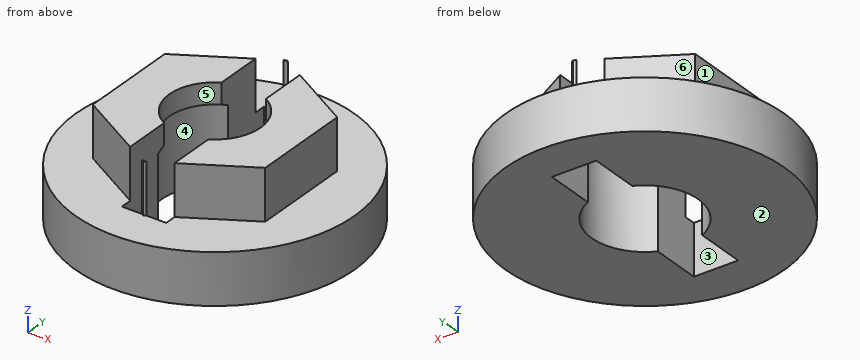
from build123d import *

# Parameters (mm, degrees)
F5_DEPTH  = 4
F4_R      = 5.5
F6_DEPTH  = 2
F7_W      = 1.75
F7_H      = 7.75
F8_DEPTH  = 5
F10_D     = 3.6
F11_D     = 4.2
F11_DEPTH = 3
F11_TIP   = 1.2618073


with BuildPart() as f5:
    # F4 (on Top) → F5 (new body)
    with BuildSketch(Plane.XY):
        Polygon((3.4, -1.9629909152), (3.4, 1.9629909152), (0, 3.9259818305), (-3.4, 1.9629909152), (-3.4, -1.9629909152), (0, -3.9259818305), align=None)
    extrude(amount=F5_DEPTH)

    # F4 (on Top) → F6 (join)
    with BuildSketch(Plane.XY):
        Circle(F4_R)
        Polygon((0, 3.9259818305), (3.4, 1.9629909152), (3.4, -1.9629909152), (0, -3.9259818305), (-3.4, -1.9629909152), (-3.4, 1.9629909152), align=None, mode=Mode.SUBTRACT)
    extrude(amount=F6_DEPTH)

    # F7 (on Top) → F8 (cut)
    with BuildSketch(Plane.XY):
        Rectangle(F7_W, F7_H)
    extrude(amount=F8_DEPTH, mode=Mode.SUBTRACT)

    # F10 (through all)
    with Locations(Plane(origin=(0, 0, 0), x_dir=(1, 0, 0), z_dir=(0, 0, -1))):
        with Locations((0, 0)):
            Hole(F10_D / 2)

    # F11
    with Locations(Plane(origin=(0, 0, 0), x_dir=(1, 0, 0), z_dir=(0, 0, -1))):
        with Locations((0, 0)):
            Hole(F11_D / 2, depth=F11_DEPTH)
            with Locations((0, 0, -(F11_DEPTH + F11_TIP / 2))):  # 118° drill point
                Cone(0, F11_D / 2, F11_TIP, mode=Mode.SUBTRACT)


solid = f5.part
Work out the finished part from the listing and answer in its coordinate system (mm). Face numbers are marked on the shaded views. A direction names the side the tool comes from. Round coordinates to 2 decimals unless told otherwise and drop trailing zeros. Write each loop counter-clockwise with the first axis right and the second up, starting at its lowest first coordinate (ties: lowest second). Pieces come first, ordered by that corner, then holes.
1) The mould has two halves that part along X. Classify the marked faces 1, 2 and 3: pulls with the +X half, pulls with the -X half, needs draft (parallel to the pull), parting line crosses it, or undercut.
2) A tool of negligible diameter and unlimited length cuts with its end or side. For the marked faces 4, 5 and 6, from which of +Z, -Z, +X, -X, +Y, -Y can it reach the whole face along a straight path? Write none if from no direction.
3) Given pin 1 Ø0.5 at (x, z) = (0.5, 2) entering from -Y; pin 2 Ø1.5 at (x, z) = (-4.5, 2) entering from -Y; pin 3 Ø1.8 at (y, z) = (2, 1.5) entering from -X, each flat-ended and moving along its own axis, determine where each tip first touches the part or whether it passes through.
4) Straight lines are drawn through the part: line 1 (Z direction, x = 3, y = -4); line 2 (Y direction, x = 1, z = 3.85); line 3 (X direction, y = -0.75, z = 3.75). For each, find the intervals that lie inside material, in ascending order.
5) A cutting plane is placed at B-B (z = 3.75). Give the vertices of the cut face in (x, y) (3 decimals), plus the area to 3 significant figures.
6) A cutting plane is placed at C-C (y = -3). Give the vertices of the cut face in (x, z) (3 decimals).
7) A cutting plane is placed at D-D (y = 2.5). Give the vertices of the cut face in (x, z) (3 decimals).
8) A cutting plane is placed at A-A (z = 0.55). Give the vertices of the cut face in (x, y) (3 decimals), plus the area to 3 significant figures.
Completed:
1. face 1: pulls with the -X half
1. face 2: needs draft
1. face 3: undercut
2. face 4: -Z
2. face 5: +Z, -Z
2. face 6: +Z, -X, +Y
3. pin 1: stops at y = -5.49
3. pin 2: stops at y = -4.02
3. pin 3: stops at x = -5.39
4. line 1: z = 0 to 2
4. line 2: y = -3.35 to -1.5, 1.5 to 3.35
4. line 3: x = -3.4 to -1.64, 1.64 to 3.4
5. outline: (-3.4, -1.963) - (-0.875, -3.421) - (-0.875, -1.573) arc R1.8 cw to (-0.875, 1.573) - (-0.875, 3.421) - (-3.4, 1.963) - close; (-0.088, -3.875) - (0, -3.926) - (0.088, -3.875) - close; (-0.088, 3.875) - (0.088, 3.875) - (0, 3.926) - close; (0.875, -3.421) - (3.4, -1.963) - (3.4, 1.963) - (0.875, 3.421) - (0.875, 1.573) arc R1.8 cw to (0.875, -1.573) - close
5. area: 23.1 mm2
6. outline: (-4.61, 0) - (-0.875, 0) - (-0.875, 4) - (-1.604, 4) - (-1.604, 2) - (-4.61, 2) - close; (0.875, 0) - (4.61, 0) - (4.61, 2) - (1.604, 2) - (1.604, 4) - (0.875, 4) - close
7. outline: (-4.899, 0) - (-0.875, 0) - (-0.875, 4) - (-2.47, 4) - (-2.47, 2) - (-4.899, 2) - close; (0.875, 0) - (4.899, 0) - (4.899, 2) - (2.47, 2) - (2.47, 4) - (0.875, 4) - close
8. outline: circle Ø11 at (0, 0); hole (-0.875, -3.875) - (0.875, -3.875) - (0.875, -1.909) arc R2.1 ccw to (0.875, 1.909) - (0.875, 3.875) - (-0.875, 3.875) - (-0.875, 1.909) arc R2.1 ccw to (-0.875, -1.909) - close
8. area: 74.7 mm2
